Here's how the part is built. I have some questions about the finished solid (model axes, mm). Face numbers are marked on the shaded views. A direction names the side the tool comes from. Coordinates: 2 decimals unless noted, no trailing zeros. Write each loop counter-clockwise with the first axis right and the second up, starting at its lowest first coordinate (ties: lowest second). Pieces come first, ordered by that corner, then holes.
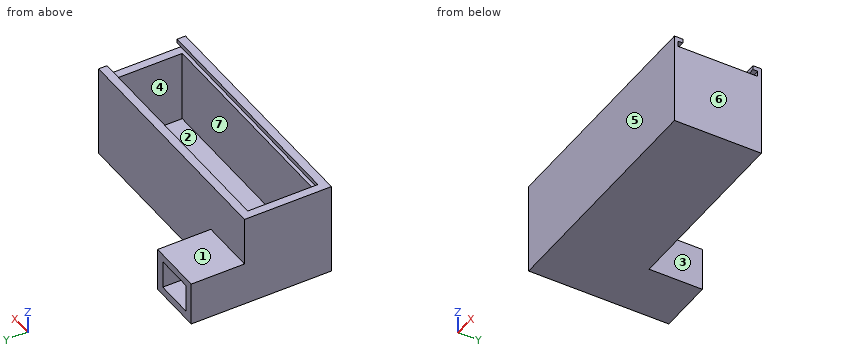
```python
from build123d import *

# Parameters (mm, degrees)
ESQUISSE1_W             = 80
ESQUISSE1_H             = 25
BOSS_EXTRU_1_DEPTH      = 4
ESQUISSE3_W             = 80
ESQUISSE3_H             = 3
BOSS_EXTRU_2_DEPTH      = 28
ESQUISSE4_W             = 28
ESQUISSE4_H             = 31
BOSS_EXTRU_3_DEPTH      = 3
ESQUISSE5_W             = 28
ESQUISSE5_H             = 31
BOSS_EXTRU_4_DEPTH      = 3
BOSS_EXTRU_5_DEPTH      = 86
ESQUISSE7_W             = 5
ESQUISSE7_H             = 3
BOSS_EXTRU_6_DEPTH      = 3
ESQUISSE8_W             = 3
ESQUISSE8_H             = 5
BOSS_EXTRU_7_DEPTH      = 25
ESQUISSE10_W            = 3
ESQUISSE10_H            = 25
BOSS_EXTRU_8_DEPTH      = 1.5
ESQUISSE11_W            = 19.800437916
ESQUISSE11_H            = 15.586484264
ESQUISSE11_W_2          = 13.800437916
ESQUISSE11_H_2          = 10
BOSS_EXTRU_9_DEPTH      = 19
ESQUISSE12_W            = 13.800437916
ESQUISSE12_H            = 10
ENL_V_MAT_EXTRU_1_DEPTH = 3


with BuildPart() as part:
    # Esquisse1 → Boss.-Extru.1 (new body)
    with BuildSketch(Plane.XY):
        with Locations((-40, 12.5)):
            Rectangle(ESQUISSE1_W, ESQUISSE1_H)
    extrude(amount=BOSS_EXTRU_1_DEPTH)

    # Esquisse3 → Boss.-Extru.2 (add)
    with BuildSketch(Plane(origin=(0, 0, 0), x_dir=(-1, 0, 0), z_dir=(0, 0, -1))):
        with Locations((40, -1.5)):
            Rectangle(ESQUISSE3_W, ESQUISSE3_H)
    boss_extru_2 = extrude(amount=-BOSS_EXTRU_2_DEPTH)

    # Symétrie1: Boss.-Extru.2 across plane
    add(boss_extru_2.mirror(Plane.ZX.offset(12.5)))

    # Esquisse4 → Boss.-Extru.3 (add)
    with BuildSketch(Plane(origin=(0, 0, 0), x_dir=(0, 0, -1), z_dir=(1, 0, 0))):
        with Locations((-14, 12.5)):
            Rectangle(ESQUISSE4_W, ESQUISSE4_H)
    extrude(amount=BOSS_EXTRU_3_DEPTH)

    # Esquisse5 → Boss.-Extru.4 (add)
    with BuildSketch(Plane.ZY.offset(80)):
        with Locations((14, 12.5)):
            Rectangle(ESQUISSE5_W, ESQUISSE5_H)
    extrude(amount=BOSS_EXTRU_4_DEPTH)

    # Esquisse6 → Boss.-Extru.5 (add)
    with BuildSketch(Plane(origin=(3, 0, 0), x_dir=(0, 0, -1), z_dir=(1, 0, 0))):
        Polygon((-31.5, 0), (-33, 0), (-33, -3), (-28, -3), (-28, 0), (-29.5, 0), (-29.5, -1.691160161), (-31.5, -1.691160161), align=None)
    boss_extru_5 = extrude(amount=-BOSS_EXTRU_5_DEPTH)

    # Esquisse7 → Boss.-Extru.6 (add)
    with BuildSketch(Plane.ZY.offset(83)):
        with Locations((30.5, -1.5)):
            Rectangle(ESQUISSE7_W, ESQUISSE7_H)
    boss_extru_6 = extrude(amount=-BOSS_EXTRU_6_DEPTH)

    # Symétrie2: Boss.-Extru.5, Boss.-Extru.6 across plane
    add(boss_extru_5.mirror(Plane.ZX.offset(12.5)))
    add(boss_extru_6.mirror(Plane.ZX.offset(12.5)))

    # Esquisse8 → Boss.-Extru.7 (add)
    with BuildSketch(Plane.XZ.offset(-25)):
        with Locations((-81.5, 30.5)):
            Rectangle(ESQUISSE8_W, ESQUISSE8_H)
    extrude(amount=BOSS_EXTRU_7_DEPTH)

    # Esquisse10 → Boss.-Extru.8 (add)
    with BuildSketch(Plane.XY.offset(28)):
        with Locations((1.5, 12.5)):
            Rectangle(ESQUISSE10_W, ESQUISSE10_H)
    extrude(amount=BOSS_EXTRU_8_DEPTH)

    # Esquisse11 → Boss.-Extru.9 (add)
    with BuildSketch(Plane(origin=(0, 28, 0), x_dir=(1, 0, 0), z_dir=(0, 1, 0))):
        with Locations((-73.099781042, -7.793242132)):
            Rectangle(ESQUISSE11_W, ESQUISSE11_H)
        with Locations((-73.131327902, -7.910815451)):
            Rectangle(ESQUISSE11_W_2, ESQUISSE11_H_2, mode=Mode.SUBTRACT)
    extrude(amount=BOSS_EXTRU_9_DEPTH)

    # Esquisse12 → Enlèv. mat.-Extru.1 (cut)
    with BuildSketch(Plane(origin=(0, 28, 0), x_dir=(1, 0, 0), z_dir=(0, 1, 0))):
        with Locations((-73.131327902, -7.910815451)):
            Rectangle(ESQUISSE12_W, ESQUISSE12_H)
    extrude(amount=-ENL_V_MAT_EXTRU_1_DEPTH, mode=Mode.SUBTRACT)


solid = part.part
```
1) Imagine slicing it at A-A on x = -49. Please give me the cut outline in (y, z), then the cut area to 3 significant figures.
Values follow:
outline: (-3, 0) - (28, 0) - (28, 33) - (25, 33) - (25, 31.5) - (26.69, 31.5) - (26.69, 29.5) - (25, 29.5) - (25, 4) - (0, 4) - (0, 29.5) - (-1.69, 29.5) - (-1.69, 31.5) - (0, 31.5) - (0, 33) - (-3, 33) - close
area: 291 mm2
2) Imagine slicing it at C-C on y = 41.5. Please give me the cut outline in (x, z), then the cut area to 3 significant figures.
Values follow:
outline: (-83, 0) - (-63.2, 0) - (-63.2, 15.59) - (-83, 15.59) - close; hole (-80.03, 2.91) - (-66.23, 2.91) - (-66.23, 12.91) - (-80.03, 12.91) - close
area: 171 mm2
3) We'd pull the mould along Y, two halves only. Please class the marked faces 4, 5, 6 and 7: pulls with the +Y half, pulls with the -Y half, needs draft (parallel to the pull), parting line crosses it, or undercut.
Values follow:
face 4: undercut
face 5: pulls with the -Y half
face 6: needs draft
face 7: undercut
4) I need wall thicknesses on probe 1 along X at (y, z) = (13, 19); probe 2 along Y at (x, z) = (-28.5, 22); probe 3 along Z at (x, y) = (-73, 37). Which ranges of each line are inside material? Lowest first, please.
Values follow:
probe 1: x = -83 to -80, 0 to 3
probe 2: y = -3 to 0, 25 to 28
probe 3: z = 0 to 2.91, 12.91 to 15.59
5) On a 3-axis mill with a long thin cutter (end or side, diameter ignored), from which of +Z, -Z, +X, -X, +Y, -Y can I reach the whole of each face in a straight line? I mean the marked faces 1, 2 and 3. Say none if no direction works.
Values follow:
face 1: +Z, +X, -X, +Y
face 2: +Z
face 3: +Z, -Z, +X, +Y
6) Will these pins go through, and if not, where does the flat tip stop? pin 1 (11 mm diameter, centred on x = -72.5, z = 7.5, fed in from +Y); pin 2 (4 mm diameter, centred on y = 41, z = 12.5, fed in from +X); pin 3 (0.8 mm diameter, centred on x = -29, z = 32.5, fed in from +Y); pin 4 (5.5 mm diameter, centred on x = -71, y = 37.5, fed in from +Z).
Values follow:
pin 1: stops at y = 47
pin 2: stops at x = -63.2
pin 3: stops at y = 28
pin 4: stops at z = 15.59
7) Imagine slicing it at D-D on y = 12. Please give me the cut outline in (x, z), then the cut area to 4 significant figures.
Values follow:
outline: (-83, 0) - (3, 0) - (3, 29.5) - (0, 29.5) - (0, 4) - (-80, 4) - (-80, 33) - (-83, 33) - close
area: 507.5 mm2
8) Imagine slicing it at B-B on z = 18. Please give me the cut outline in (x, y), then the cut area to 3 significant figures.
Values follow:
outline: (-83, -3) - (3, -3) - (3, 28) - (-83, 28) - close; hole (-80, 0) - (0, 0) - (0, 25) - (-80, 25) - close
area: 666 mm2
